Can you work these out from the drawing? Everything is in mm from the part's minimum corner. A direction names the side the tool comes from. Coordinates: 2 decimals unless noted, no trailing zeros. Loops run counter-clockwise (first coordinate to the right, second up) from the corner with the lowest first, then second, coordinate; pieces in that order, holes last.
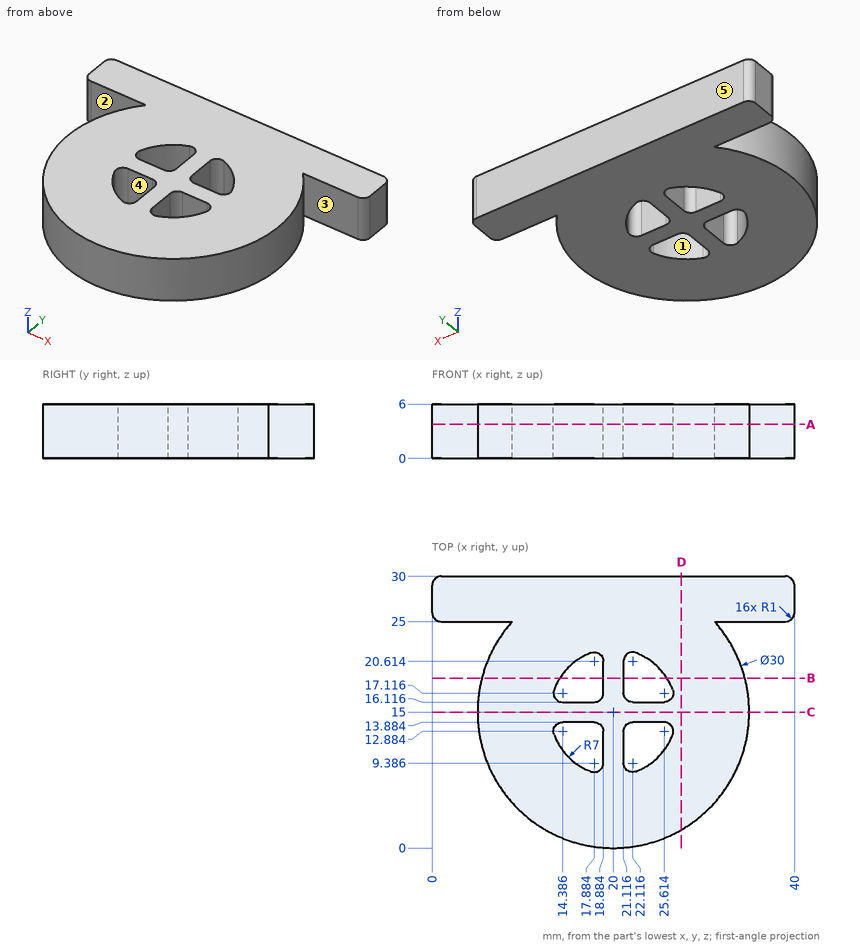
Item 1: Suppose I cut it at D-D, the plane x = 27.5. Please give me the cut outline in (y, z).
Results are:
outline: (2.01, 0) - (30, 0) - (30, 6) - (2.01, 6) - close
Item 2: We'd pull the mould along X, two halves only. Please class the marked faces 4 and 5: +X half, -X half, draft (parallel to the pull), parting line (faces both ways), or undercut.
Results are:
face 4: undercut
face 5: draft
Item 3: Suppose I cut it at B-B, the plane y = 18.75. Please give me the cut outline in (x, z).
Results are:
outline: (5.48, 0) - (14.09, 0) - (14.09, 6) - (5.48, 6) - close; (18.88, 0) - (21.12, 0) - (21.12, 6) - (18.88, 6) - close; (25.91, 0) - (34.52, 0) - (34.52, 6) - (25.91, 6) - close
Item 4: On a 3-axis mill with a long thin cutter (end or side, diameter ignored), from which of +Z, -Z, +X, -X, +Y, -Y can I reach the whole of each face in a straight line? I mean the marked faces 1, 2 and 3. Say none if no direction works.
Results are:
face 1: +Z, -Z
face 2: +Z, -Z, -X
face 3: +Z, -Z, +X
Item 5: Suppose I cut it at C-C, the plane y = 15. Please give me the cut outline in (x, z).
Results are:
outline: (5, 0) - (35, 0) - (35, 6) - (5, 6) - close
Item 6: I'm going to push flat-ended pins straight in: P1, Ø1.7, axis at y = 11, z = 3.5, coming from the -X side (1 decimal); P2, Ø1, axis at y = 19.5, z = 2, coming from the +X side; P3, Ø2, axis at x = 22, z = 3, coming from the -Y side. Where does each tip first touch, or does it pass through?
Results are:
P1: stops at x = 5.3
P2: stops at x = 34.46
P3: stops at y = 0.03
Item 7: I need wall thicknesses on line 1 along X through (y, z) = (19.5, 3.35) (1 decimal); line 2 along X through (y, z) = (19.75, 3.45) (1 decimal); line 3 along Y through (x, z) = (33, 3.1) (1 decimal). Which ranges of each line are inside material? Lowest first, please.
Results are:
line 1: x = 5.7 to 14.6, 18.9 to 21.1, 25.4 to 34.3
line 2: x = 5.8 to 14.9, 18.9 to 21.1, 25.1 to 34.2
line 3: y = 7.5 to 22.5, 25 to 30
Item 8: Suppose I cut it at A-A, the plane z = 3.75. Count the separate pieces of the cut face and the enclosed holes in it, plus the area to 3 significant figures.
Results are:
separate pieces: 1
enclosed holes: 4
area: 736 mm2
